from build123d import *

# Parameters (mm, degrees)
RESSALTO_EXTRUS_O1_DEPTH          = 20.4
REBAIXO_PARA_SHCS_M61_D           = 6.6
REBAIXO_PARA_SHCS_M61_CBORE_D     = 11
REBAIXO_PARA_SHCS_M61_CBORE_DEPTH = 6
ESBO_O14_R                        = 17.5
RESSALTO_EXTRUS_O2_DEPTH          = 10.4
FURO_ROSCADO_DE_M5X0_81_D         = 4.2
FURO_ROSCADO_DE_M5X0_81_DEPTH     = 14
FURO_ROSCADO_DE_M5X0_81_TIP       = 1.2618073


with BuildPart() as part:
    # Esboço1 → Ressalto-extrusão1 (new body)
    with BuildSketch(Plane.XY):
        with BuildLine():
            Line((-23.5, 110), (100, 110))
            Line((100, 110), (100, -110))
            Line((100, -110), (-23.5, -110))
            Line((-23.5, -110), (-23.5, -18.648056199))
            ThreePointArc((-23.5, -18.648056199), (30, 0), (-23.5, 18.648056199))
            Line((-23.5, 18.648056199), (-23.5, 110))
        make_face()
    extrude(amount=RESSALTO_EXTRUS_O1_DEPTH)

    # Rebaixo para SHCS M61 (through all)
    with Locations(Plane.XY.offset(20.4)):
        with Locations((93.5, 100), (93.5, 0), (93.5, -100)):
            CounterBoreHole(REBAIXO_PARA_SHCS_M61_D / 2, REBAIXO_PARA_SHCS_M61_CBORE_D / 2, REBAIXO_PARA_SHCS_M61_CBORE_DEPTH)

    # Esboço14 → Ressalto-extrusão2 (add)
    with BuildSketch(Plane.XY.offset(10)):
        with BuildLine():
            Line((-23.5, -18.648056199), (-23.5, 18.648056199))
            ThreePointArc((-23.5, 18.648056199), (30, 0), (-23.5, -18.648056199))
        make_face()
        Circle(ESBO_O14_R, mode=Mode.SUBTRACT)
    extrude(amount=RESSALTO_EXTRUS_O2_DEPTH)

    # Furo roscado de M5x0.81
    with Locations(Plane.XY.offset(20.4)):
        with Locations((30, 100.827560784), (93.5, 60), (93.5, -60), (30, -102.194888391)):
            Hole(FURO_ROSCADO_DE_M5X0_81_D / 2, depth=FURO_ROSCADO_DE_M5X0_81_DEPTH)
            with Locations((0, 0, -(FURO_ROSCADO_DE_M5X0_81_DEPTH + FURO_ROSCADO_DE_M5X0_81_TIP / 2))):  # 118° drill point
                Cone(0, FURO_ROSCADO_DE_M5X0_81_D / 2, FURO_ROSCADO_DE_M5X0_81_TIP, mode=Mode.SUBTRACT)


solid = part.part
Source: CAD feature listing. Evaluate the final solid. Frame: model axes, mm. A direction names the side the tool comes from. Coordinates: 2 decimals unless noted, no trailing zeros. Loops run counter-clockwise (first coordinate to the right, second up) from the corner with the lowest first, then second, coordinate; pieces in that order, holes last. Notation, with made-up numbers: M 83,-2.5 L 134,-2.5 A20 ccw 134,11.5 Z; hole C 34,-1 d3. An arc over 180 degrees is marked long. Answer in a Markdown table with one row per item.
Q1. Section A-A on x = 2.5. Return the cut outline in (y, z).
Answers below:
| item | result |
|---|---|
| outline | M -110,0 L -29.9,0 L -29.9,10 L -17.32,10 L -17.32,20.4 L -110,20.4 Z; M 17.32,10 L 29.9,10 L 29.9,0 L 110,0 L 110,20.4 L 17.32,20.4 Z |
Q2. Section D-D on x = 21. Return the cut outline in (y, z), plus the area to 3 significant figures.
Answers below:
| item | result |
|---|---|
| outline | M -110,0 L -21.42,0 L -21.42,10 L 21.42,10 L 21.42,0 L 110,0 L 110,20.4 L -110,20.4 Z |
| area | 4,060 mm^2 |
Q3. Set-up query: faces 1 (the cylindrical face through (29.98, -1.04, 4.93)), 2 (the cylindrical face through (88, 0, 17)), 3 (the flat face through (39, 2, 20.4)). Return all of +Z, -Z, +X, -X, +Y, -Y with unobstructed straight access to the full face (end or side cutting, diameter ignored); none if empty.
Answers below:
| item | result |
|---|---|
| face 1 | -Z |
| face 2 | +Z |
| face 3 | +Z, +X, -X, +Y, -Y |
Q4. First-contact query: pin 1 (2.5 mm diameter, centred on x = 30, y = 100.83, fed in from +Z); pin 2 (3.5 mm diameter, centred on x = 30, y = -102.19, fed in from +Z); pin 3 (3.5 mm diameter, centred on x = 96, y = -98, fed in from +Z). Flat tips, straight axial feed; report the tip coordinate or a pass-through.
Answers below:
| item | result |
|---|---|
| pin 1 | stops at z = 5.89 |
| pin 2 | stops at z = 6.19 |
| pin 3 | stops at z = 14.4 |
Q5. Section C-C on z = 3. Return the cut outline in (x, y), plus the area to 3 significant figures.
Answers below:
| item | result |
|---|---|
| outline | M -23.5,-110 L 100,-110 L 100,110 L -23.5,110 L -23.5,18.65 A30 cw long -23.5,-18.65 Z; hole C 93.5,-100 d6.6; hole C 93.5,0 d6.6; hole C 93.5,100 d6.6 |
| area | 24,400 mm^2 |
Q6. Section B-B on y = 13. Return the cut outline in (x, z).
Answers below:
| item | result |
|---|---|
| outline | M -23.5,10 L -11.72,10 L -11.72,20.4 L -23.5,20.4 Z; M 11.72,10 L 27.04,10 L 27.04,0 L 100,0 L 100,20.4 L 11.72,20.4 Z |
Q7. Ray query, probe 1 along Y at (x, z) = (93.5, 5); probe 2 along Y at (x, z) = (93.5, 17.75); probe 3 along Y at (x, z) = (93.5, 10). Return the intervals inside material, ascending. Write a range as from..to.
Answers below:
| item | result |
|---|---|
| probe 1 | y = -110..-103.3, -96.7..-3.3, 3.3..96.7, 103.3..110 |
| probe 2 | y = -110..-105.5, -94.5..-62.1, -57.9..-5.5, 5.5..57.9, 62.1..94.5, 105.5..110 |
| probe 3 | y = -110..-103.3, -96.7..-62.1, -57.9..-3.3, 3.3..57.9, 62.1..96.7, 103.3..110 |
Q8. Draft query along X for faces 4 (the flat face through (37, 110, 10)), 5 (the conical face through (93.7, -59.69, 5.36)), 6 (the flat face through (-23.5, -2, 12)). Return one class per face: pulls with the +X half, pulls with the -X half, needs draft (parallel to the pull), parting line crosses it, or undercut.
Answers below:
| item | result |
|---|---|
| face 4 | needs draft |
| face 5 | undercut |
| face 6 | pulls with the -X half |
